Check sheet for the modelled part. Datum: model origin and axes. Units: mm. Give positions to 0.01 mm unless a question says otherwise; leave off trailing zeros. Write each loop counter-clockwise with the first axis right and the second up, starting at its lowest first coordinate (ties: lowest second). Pieces come first, ordered by that corner, then holes. Notation, with made-up numbers: (-37.5, 23.25) -> (-7.5, 23.25) arc R9 ccw to (-7.5, 28.25) -> close; hole circle Ø5 at (1.25, 24.5). An arc over 180 degrees is marked (long way). Return JSON: item names as keys, results as strings.
from build123d import *

# Parameters (mm, degrees)
F0_R     = 23
F0_R_2   = 20
F1_DEPTH = 20
F2_R     = 23
F3_DEPTH = 3
F4_R     = 1
F5_R     = 1
F6_R     = 1


with BuildPart() as f1:
    # F0 (on Top) → F1 (new body)
    with BuildSketch(Plane.XY):
        Circle(F0_R)
        Circle(F0_R_2, mode=Mode.SUBTRACT)
    extrude(amount=F1_DEPTH)

    # F2 (on Top) → F3 (join)
    with BuildSketch(Plane.XY):
        Circle(F2_R)
    extrude(amount=F3_DEPTH)

    # F4
    f4_edges = [f1.edges().sort_by_distance(p)[0] for p in [
        (-20, 0, 20),
    ]]
    fillet(f4_edges, radius=F4_R)

    # F5
    f5_edges = [f1.edges().sort_by_distance(p)[0] for p in [
        (-23, 0, 20),
    ]]
    fillet(f5_edges, radius=F5_R)

    # F6
    f6_edges = [f1.edges().sort_by_distance(p)[0] for p in [
        (-20, 0, 3),
    ]]
    fillet(f6_edges, radius=F6_R)


solid = f1.part
(1) Thickness scan on L1, parallel to Y at x = 0, z = 15; L2, parallel to Z at x = 3, y = 16.5; L3, parallel to X at y = -12, z = 5.5. Record the ranges inside material, lowest first.
Reply:
{"L1": "-23 to -20, 20 to 23", "L2": "0 to 3", "L3": "-19.62 to -16, 16 to 19.62"}
(2) Cross-section at B-B on z = 11.5. Enter the section's corners in (x, y), then the cut area to 3 significant figures.
Reply:
{"outline": "circle Ø46 at (0, 0); hole circle Ø40 at (0, 0)", "area": "405 mm^2"}
(3) Release check for a two-part mould opening along X. For faces 1 (the cylindrical face through (-2.994, 22.804, 9.367)), 2 (the flat face through (0, 0, 0)), 3 (the flat face through (0, 0, 3)) record: pulls with the +X half, pulls with the -X half, needs draft (parallel to the pull), parting line crosses it, or undercut.
Reply:
{"face 1": "parting line crosses it", "face 2": "needs draft", "face 3": "undercut"}
(4) Cross-section at A-A on x = 0. Enter the section's corners in (y, z).
Reply:
{"outline": "(-23, 0) -> (23, 0) -> (23, 19) arc R1 ccw to (22, 20) -> (21, 20) arc R1 ccw to (20, 19) -> (20, 4) arc R1 cw to (19, 3) -> (-19, 3) arc R1 cw to (-20, 4) -> (-20, 19) arc R1 ccw to (-21, 20) -> (-22, 20) arc R1 ccw to (-23, 19) -> close"}
(5) Depth check by flat-ended pin: pin 1 Ø5 at (x, z) = (-3, 15) entering from +Y; pin 2 Ø8 at (y, z) = (11, 3) entering from +X; pin 3 Ø4 at (y, z) = (17.5, 9) entering from -X. Enter the tip coordinate at first touch or a pass-through.
Reply:
{"pin 1": "y = 22.99", "pin 2": "x = 21.91", "pin 3": "x = -16.99"}
